```python
from build123d import *

# Parameters (mm, degrees)
EXTRUDE_1_DEPTH     = 3.8
CUT_EXTRUDE_1_DEPTH = 5.6
SKETCH_4_R          = 0.3
EXTRUDE_2_DEPTH     = 3
EXTRUDE_2_2_DEPTH   = 3
SKETCH_4_2_R        = 0.3
EXTRUDE_3_DEPTH     = 0.5


with BuildPart() as part:
    # Sketch 2 → Extrude 1 (new body)
    with BuildSketch(Plane.XY):
        Polygon((2.54, -2), (0, -2), (0, 0), (0, 2), (2.54, 2), (5.08, 2), (5.08, 0), (5.08, -2), align=None)
    extrude(amount=EXTRUDE_1_DEPTH)

    # Sketch 3 → Cut-Extrude 1 (cut)
    with BuildSketch(Plane(origin=(0, 2, 0), x_dir=(-1, 0, 0), z_dir=(0, 1, 0))):
        Polygon((0, 0), (0, 0.5), (-2, 0.5), (-2.2, 0), align=None)
        Polygon((-2.88, 0), (-5.08, 0), (-5.08, 0.5), (-3.08, 0.5), align=None)
    extrude(amount=-CUT_EXTRUDE_1_DEPTH, mode=Mode.SUBTRACT)



with BuildPart() as body_2:
    # Sketch 4 → Extrude 2 (new body)
    with BuildSketch(Plane.XY):
        Circle(SKETCH_4_R)
    extrude(amount=-EXTRUDE_2_DEPTH)


with BuildPart() as body_3:
    # Sketch 4 → Extrude 2 2 (new body)
    with BuildSketch(Plane.XY):
        with Locations(Location((5.08, 0, 0), (0, 0, 180))):
            Circle(SKETCH_4_R)
    extrude(amount=-EXTRUDE_2_2_DEPTH)


with BuildPart() as part_1:
    add(part.part)

    add(body_2.part)  # Extrude 3 merges body 2

    add(body_3.part)  # Extrude 3 merges body 3
    # Sketch 4_2 → Extrude 3 (add)
    with BuildSketch(Plane.XY):
        with Locations(Location((0, 0, 0), (0, 0, 90))):
            Circle(SKETCH_4_2_R)
        with Locations(Location((5.08, 0, 0), (0, 0, 90))):
            Circle(SKETCH_4_2_R)
    extrude(amount=EXTRUDE_3_DEPTH)


solid = part_1.part
```
Work out the finished part from the listing and answer in its coordinate system (mm). Give positions to 0.01 mm unless a question says otherwise; leave off trailing zeros. Order: outer loops, then holes, each group sorted by start corner. A loop starts at its lowest first (then second) coordinate and runs counter-clockwise, first axis right, second up. Notation, with made-up numbers: M -29.5,49.25 L 0.5,49.25 A25 cw 0.5,72.25 Z; hole C 86.5,76 d3. An arc over 180 degrees is marked long. Return JSON: item names as keys, results as strings.
1) Section D-D, the plane z = 1 is taken. Write down the section's boundary in (x, y).
Resolved:
{"outline": "M 0,-2 L 5.08,-2 L 5.08,2 L 0,2 Z"}
2) Each of these flat-tipped pins is pushed along its axis until it touches: pin 1 (0.6 mm diameter, centred on x = 4, y = 0, fed in from -Z); pin 2 (2 mm diameter, centred on x = 1, y = 0, fed in from -Z); pin 3 (1 mm diameter, centred on y = 1, z = 3, fed in from -X); pin 4 (0.5 mm diameter, centred on x = 2.5, y = -1, fed in from -Z). Where does it stop, or does it pass through?
Resolved:
{"pin 1": "z = 0.5", "pin 2": "z = -3", "pin 3": "x = 0", "pin 4": "z = 0"}
3) Section C-C, the plane x = 4.7 is taken. Write down the section's boundary in (y, z).
Resolved:
{"outline": "M -2,0.5 L 2,0.5 L 2,3.8 L -2,3.8 Z"}
4) Section A-A, the plane y = -0.4 is taken. Write down the section's boundary in (x, z).
Resolved:
{"outline": "M 0,0.5 L 2,0.5 L 2.2,0 L 2.88,0 L 3.08,0.5 L 5.08,0.5 L 5.08,3.8 L 0,3.8 Z"}
5) Straight lines are drawn through the part: line 1 along X through (y, z) = (-0.5, 2.25); line 2 along Z through (x, y) = (3, -1.7); line 3 along Z through (x, y) = (2.8, 0.55). For each, find the intervals that lie inside material, in ascending order. Write a range as [from, to].
Resolved:
{"line 1": "[0, 5.08]", "line 2": "[0.3, 3.8]", "line 3": "[0, 3.8]"}
6) Section B-B, the plane z = -1 is taken. Write down the section's boundary in (x, y), plus the area to 3 significant figures.
Resolved:
{"outline": "C 0,0 d0.6; C 5.08,0 d0.6", "area": "0.565 mm^2"}
